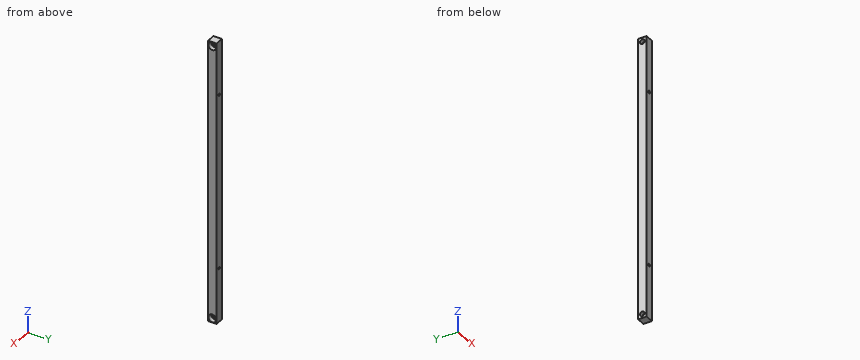
from build123d import *

# Parameters (mm, degrees)
IZIM1_W                     = 15
IZIM1_H                     = 15
Y_KSEKLIK_EKSTR_ZYON1_DEPTH = 252.5
DELIK1_D                    = 8.5
DELIK1_CBORE_D              = 14
DELIK1_CBORE_DEPTH          = 8
M5_DI_LI_DELIK1_D           = 4.2
M5_DI_LI_DELIK1_DEPTH       = 24
M5_DI_LI_DELIK1_CSINK_D     = 5.05
M5_DI_LI_DELIK1_CSINK_ANGLE = 90
M5_DI_LI_DELIK1_TIP         = 1.2618073


with BuildPart() as part:
    # Çizim1 → Yükseklik-Ekstrüzyon1 (new, symmetric)
    with BuildSketch(Plane.XY):
        Rectangle(IZIM1_W, IZIM1_H)
    extrude(amount=Y_KSEKLIK_EKSTR_ZYON1_DEPTH, both=True)

    # Delik1 (through all)
    with Locations(Plane(origin=(7.5, 0, -245), x_dir=(0, 0, 1), z_dir=(1, 0, 0))):
        with Locations((0, 0)):
            delik1 = CounterBoreHole(DELIK1_D / 2, DELIK1_CBORE_D / 2, DELIK1_CBORE_DEPTH)

    # Aynalama1: Delik1 across plane
    add(delik1.mirror(Plane.XY), mode=Mode.SUBTRACT)

    # M5 Dişli Delik1
    with Locations(Plane(origin=(0, -7.5, 0), x_dir=(-1, 0, 0), z_dir=(0, -1, 0))):
        with Locations((0, 155.996395214), (0, -155.996395214)):
            CounterSinkHole(M5_DI_LI_DELIK1_D / 2, M5_DI_LI_DELIK1_CSINK_D / 2, depth=M5_DI_LI_DELIK1_DEPTH, counter_sink_angle=M5_DI_LI_DELIK1_CSINK_ANGLE)
            with Locations((0, 0, -(M5_DI_LI_DELIK1_DEPTH + M5_DI_LI_DELIK1_TIP / 2))):  # 118° drill point
                Cone(0, M5_DI_LI_DELIK1_D / 2, M5_DI_LI_DELIK1_TIP, mode=Mode.SUBTRACT)


solid = part.part
Work out the finished part from the listing and answer in its coordinate system (mm). Give positions to 0.01 mm unless a question says otherwise; leave off trailing zeros. Loops run counter-clockwise (first coordinate to the right, second up) from the corner with the lowest first, then second, coordinate; pieces in that order, holes last. Notation, with made-up numbers: (64, -7) -> (74, -7) arc R22 ccw to (74, 21) -> close; hole circle Ø5 at (69, 86.25). An arc over 180 degrees is marked (long way). Use a Markdown table: item, result. Add a question column.
1. Section A-A on z = 245 is taken. Determine the outline of the cut face in (x, y), and give its area (3 significant figures).
2. Section B-B on y = 0 is taken. Determine the outline of the cut face in (x, z), and give its area (3 significant figures).
3. Find the intervals of material crossed by probe 1 along Z at (x, y) = (6.75, -0.5); probe 2 along Z at (x, y) = (3.25, 3); probe 3 along Y at (x, z) = (3.5, -245), in increasing order.
Results below:
| question | item | result |
|---|---|---|
| 1 | outline | (-7.5, -7.5) -> (7.5, -7.5) -> (7.5, -7) -> (-0.5, -7) -> (-0.5, -4.25) -> (-7.5, -4.25) -> close; (-7.5, 4.25) -> (-0.5, 4.25) -> (-0.5, 7) -> (7.5, 7) -> (7.5, 7.5) -> (-7.5, 7.5) -> close |
| 1 | area | 53.5 mm^2 |
| 2 | outline | (-7.5, -252.5) -> (7.5, -252.5) -> (7.5, -252) -> (-0.5, -252) -> (-0.5, -249.25) -> (-7.5, -249.25) -> close; (-7.5, -240.75) -> (-0.5, -240.75) -> (-0.5, -238) -> (7.5, -238) -> (7.5, 238) -> (-0.5, 238) -> (-0.5, 240.75) -> (-7.5, 240.75) -> close; (-7.5, 249.25) -> (-0.5, 249.25) -> (-0.5, 252) -> (7.5, 252) -> (7.5, 252.5) -> (-7.5, 252.5) -> close; hole circle Ø4.2 at (0, -156); hole circle Ø4.2 at (0, 156) |
| 2 | area | 7,200 mm^2 |
| 3 | probe 1 | z = -252.5 to -251.98, -238.02 to 238.02, 251.98 to 252.5 |
| 3 | probe 2 | z = -252.5 to -251.32, -238.68 to 238.68, 251.32 to 252.5 |
| 3 | probe 3 | y = -7.5 to -7, 7 to 7.5 |
